```python
from build123d import *

# Parameters (mm, degrees)
ESBO_O1_W             = 20
ESBO_O1_H             = 20
ESBO_O1_W_2           = 16
ESBO_O1_H_2           = 16
EXTRUS_O_FINA1_DEPTH  = 337
ESBO_O2_R             = 2.5
CORTE_EXTRUS_O1_DEPTH = 339.18486069
ESBO_O3_R             = 2.6
ESBO_O3_R_2           = 2.8
CORTE_EXTRUS_O2_DEPTH = 339.18486069
ESBO_O4_R             = 2.5
CORTE_EXTRUS_O3_DEPTH = 339.18486069


with BuildPart() as part:
    # Esboço1 → Extrusão-Fina1 (new body)
    with BuildSketch(Plane(origin=(0, 0, 0), x_dir=(1, 0, 0), z_dir=(0, 1, 0))):
        with Locations((10, 10)):
            Rectangle(ESBO_O1_W, ESBO_O1_H)
        with Locations((10, 10)):
            Rectangle(ESBO_O1_W_2, ESBO_O1_H_2, mode=Mode.SUBTRACT)
    extrude(amount=EXTRUS_O_FINA1_DEPTH)

    # Esboço2 → Corte-extrusão1 (cut, through all)
    with BuildSketch(Plane.ZY):
        with Locations((-10, 35)):
            Circle(ESBO_O2_R)
        with Locations((-10, 10)):
            Circle(ESBO_O2_R)
    extrude(amount=-CORTE_EXTRUS_O1_DEPTH, mode=Mode.SUBTRACT)

    # Esboço3 → Corte-extrusão2 (cut, through all)
    with BuildSketch(Plane(origin=(0, 0, -20), x_dir=(-1, 0, 0), z_dir=(0, 0, -1))):
        with Locations((-10, 310)):
            Circle(ESBO_O3_R)
        with Locations((-10, 332)):
            Circle(ESBO_O3_R_2)
    extrude(amount=-CORTE_EXTRUS_O2_DEPTH, mode=Mode.SUBTRACT)

    # Esboço4 → Corte-extrusão3 (cut, through all)
    with BuildSketch(Plane(origin=(20, 0, 0), x_dir=(0, 0, -1), z_dir=(1, 0, 0))):
        with Locations((10, 321)):
            Circle(ESBO_O4_R)
    extrude(amount=-CORTE_EXTRUS_O3_DEPTH, mode=Mode.SUBTRACT)


solid = part.part
```
CAD build for the part. Positions are in the model's coordinates, mm. A direction names the side the tool comes from. Round coordinates to 2 decimals unless told otherwise and drop trailing zeros. Write each loop counter-clockwise with the first axis right and the second up, starting at its lowest first coordinate (ties: lowest second). Pieces come first, ordered by that corner, then holes. Notation, with made-up numbers: (34.25, -23.5) - (93.25, -23.5) arc R16 ccw to (93.25, -12.5) - close; hole circle Ø3 at (-35.5, 79). An arc over 180 degrees is marked (long way). Write item = value, one per line. Start each with the question number.
Q1. Mould opens along Z. For faces 1 (the flat face through (1, 337, -10)), 2 (the flat face through (10, 166, -2)), 3 (the flat face through (10, 166, -18)), 4 (the flat face through (10, 166, 0)) say: pulls with the +Z half, pulls with the -Z half, needs draft (parallel to the pull), parting line crosses it, or undercut.
Q2. Which spindle directions (+Z, -Z, +X, -X, +Y, -Y) get a long thin tool onto all of the face, cutting with end or side? Do faces 5 (the flat face through (18, 166, -10)), 6 (the flat face through (20, 166, -10)). Say none if no direction does.
Q3. Probe L1, parallel to Y at x = 1.65, z = -10; L2, parallel to Y at x = 10, z = -19.2; L3, parallel to X at y = 310, z = -18.35. List the from-to ranges inside material, lowest first. Write a range as from..to.
Q4. Band-saw the part on B-B (y = 42). Give the cut face in (x, z), then the cut area to 3 significant figures.
Q5. Band-saw the part on A-A (z = -4.75). Give the cut face in (x, y).
Answers below:
q1.face_1 = needs draft
q1.face_2 = undercut
q1.face_3 = undercut
q1.face_4 = pulls with the +Z half
q2.face_5 = +Y, -Y
q2.face_6 = +Z, -Z, +X, +Y, -Y
q3.L1 = 0..7.5, 12.5..32.5, 37.5..318.5, 323.5..337
q3.L2 = 0..307.4, 312.6..329.2, 334.8..337
q3.L3 = 0..7.4, 12.6..20
q4.outline = (0, -20) - (20, -20) - (20, 0) - (0, 0) - close; hole (2, -18) - (18, -18) - (18, -2) - (2, -2) - close
q4.area = 144 mm2
q5.outline = (0, 0) - (2, 0) - (2, 337) - (0, 337) - close; (18, 0) - (20, 0) - (20, 337) - (18, 337) - close
